The figure shows three views and two pictorial views of one solid part (mm, origin at its lowest corner). Answer the questions. A direction names the side the tool comes from. Coordinates: 2 decimals unless noted, no trailing zeros. Write each loop counter-clockwise with the first axis right and the second up, starting at its lowest first coordinate (ties: lowest second). Pieces come first, ordered by that corner, then holes. Notation, with made-up numbers: M 50,66 L 84,66 A26 cw 84,93 Z; hole C 30.25,78 d9. An arc over 180 degrees is marked long. Answer as CSV lines item,"result".
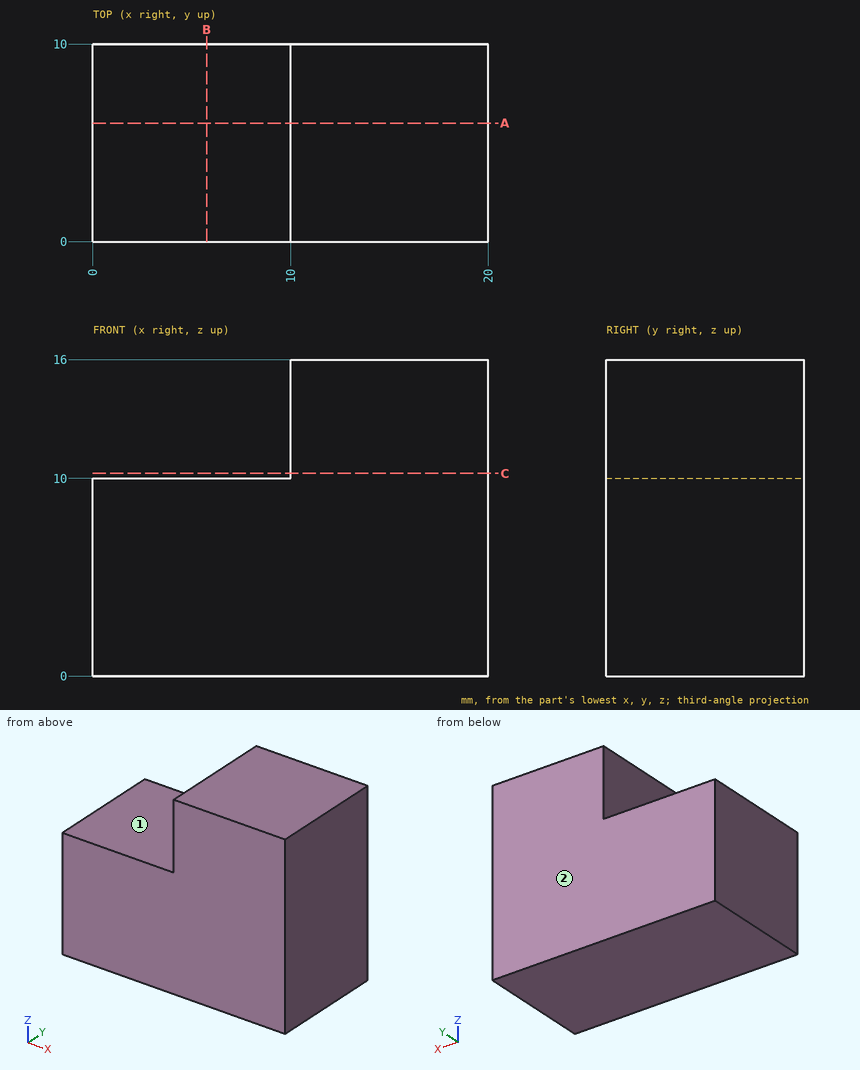
Q1. Find section A-A (y = 6). Give the vertices of the cut face in (x, z), and give its area (3 significant figures).
Output:
outline,"M 0,0 L 20,0 L 20,16 L 10,16 L 10,10 L 0,10 Z"
area,"260 mm2"
Q2. Straight lines are drawn through the part: line 1 (Z direction, x = 9.25, y = 7.25); line 2 (X direction, y = 9, z = 15). For each, find the intervals that lie inside material, in ascending order.
Output:
line 1,"0 to 10"
line 2,"10 to 20"
Q3. Flat-ended cylindrical pins translate along their axes: pin 1 Ø3 at (y, z) = (3.5, 12.5) entering from -X; pin 2 Ø5 at (x, y) = (5.5, 5.5) entering from +Z. Find the tip coordinate at first contact, or state that the pin passes through.
Output:
pin 1,"x = 10"
pin 2,"z = 10"
Q4. For the marked faces 1 and 2, determine the directions among +Z, -Z, +X, -X, +Y, -Y from which every point of the face is accessible in a straight line to the end or side of a thin tool.
Output:
face 1,"+Z, -X, +Y, -Y"
face 2,"+Z, -Z, +X, -X, +Y"
Q5. Find section C-C (z = 10.25). Give the vertices of the cut face in (x, y).
Output:
outline,"M 10,0 L 20,0 L 20,10 L 10,10 Z"
Q6. Find section B-B (x = 5.75). Give the vertices of the cut face in (y, z), and give its area (3 significant figures).
Output:
outline,"M 0,0 L 10,0 L 10,10 L 0,10 Z"
area,"100 mm2"
